Autodesk Inventor part; units mm, degrees
ref_plane "Work Plane1" through (0, 5, 0) normal (0, 1, 0) x (1, 0, 0)
ref_plane "Work Plane3" through (0, 15.4, 0) normal (0, 1, 0) x (1, 0, 0)
ref_plane "YZ Plane" through (0, 0, 0) normal (1, 0, 0) x (0, 1, 0)
sketch "Sketch1" plane through (0, 0, 0) normal (0, 1, 0) x (-1, 0, 0)
  circle A0 centre (0, 0) radius 88.9
  dimension "d0" = 177.8
extrude "Extrusion1" add sketch "Sketch1" along normal blind 25.4
sketch "Sketch2" plane through (0, 25.4, 0) normal (0, 1, 0) x (1, 0, 0)
  circle A0 centre (0, 0) radius 87.4
  line L0 (0, 0) -> (-10.8342, 88.2374)
  circle A1 centre (0, 0) radius 88.9
  line L1 (0, 0) -> (10.8342, 88.2374)
  circle A2 centre (0, 0) radius 34.925
  line L2 (0, 0) -> (0, 88.9)
  circle A3 centre (0, 0) radius 41.275
  point P0 (-4.2563, 34.6647)
  point P1 (4.2563, 34.6647)
  point P2 (10.6514, 86.7485)
  point P3 (-10.6514, 86.7485)
  point P4 (-5.0302, 40.9673)
  point P5 (5.0302, 40.9673)
  dimension "d3" = 174.8
  dimension "d4" = 69.85
  dimension "d10" = 14
  dimension "d11" = 7
  dimension "d45" = 82.55
extrude "Extrusion2" cut sketch "Sketch2" against normal blind 25.4 contours L1 A3 L2 A0 | A0 L2 A3 L0
pattern_circular "Circular Pattern1" count 22 over 360 about axis through (0, 0, 0) along (0, 1, 0) of "Extrusion2"
sketch "Sketch4" plane through (0, 25.4, 0) normal (0, 1, 0) x (1, 0, 0)
  circle A0 centre (0, 0) radius 32.425
  dimension "d16" = 64.85
extrude "Extrusion3" cut sketch "Sketch4" against normal blind 20.4
ref_plane "Work Plane1" through (0, 5, 0) normal (0, 1, 0) x (1, 0, 0)
sketch "Sketch5" plane through (0, 5, 0) normal (0, 1, 0) x (1, 0, 0)
  line L0 (0, 0) -> (0, 25)
  line L1 (0, 0) -> (-25, 0)
  line L2 (0, 0) -> (0, -25)
  line L3 (0, 0) -> (25, 0)
  line L4 (25, 0) -> (25, -9)
  line L5 (0, -25) -> (9, -25)
  line L6 (9, -25) -> (9, -9)
  line L7 (9, -9) -> (25, -9)
  line L8 (0, -25) -> (-9, -25)
  line L9 (-9, -25) -> (-9, -9)
  line L10 (-9, -9) -> (-25, -9)
  line L11 (-25, -9) -> (-25, 0)
  line L12 (-25, 0) -> (-25, 9)
  line L13 (-25, 9) -> (-9, 9)
  line L14 (-9, 9) -> (-9, 25)
  line L15 (-9, 25) -> (0, 25)
  line L16 (9, 25) -> (0, 25)
  line L17 (9, 25) -> (9, 9)
  line L18 (9, 9) -> (25, 9)
  line L19 (25, 9) -> (25, 0)
  dimension "d65" = 25
  dimension "d66" = 25
  dimension "d67" = 25
  dimension "d68" = 25
  dimension "d69" = 9
  dimension "d70" = 9
  dimension "d71" = 9
  dimension "d72" = 9
  dimension "d85" = 9
  dimension "d86" = 9
  dimension "d87" = 9
  dimension "d88" = 9
extrude "Extrusion4" add sketch "Sketch5" along normal blind 15
ref_plane "Work Plane3" through (0, 15.4, 0) normal (0, 1, 0) x (1, 0, 0)
sketch "Sketch21" plane through (0, 25.4, 0) normal (0, 1, 0) x (1, 0, 0)
  circle A0 centre (0, 0) radius 32.425
  circle A1 centre (0, 0) radius 37.425
  dimension "d51" = 64.85
  dimension "d52" = 74.85
extrude "Extrusion8" cut sketch "Sketch21" against normal blind 2
sketch "Sketch23" plane through (0, 0, 0) normal (0, -1, 0) x (1, 0, 0)
  circle A0 centre (0, 0) radius 11
  dimension "d60" = 22
extrude "Extrusion10" cut sketch "Sketch23" against normal blind 7
sketch "Sketch7" plane through (0, 15.4, 0) normal (0, 1, 0) x (1, 0, 0)
  line L0 (-6, 6) -> (6, 6)
  line L1 (6, 6) -> (6, -6)
  line L2 (6, -6) -> (-6, -6)
  line L3 (-6, -6) -> (-6, 6)
  line L4 (-15, 15) -> (15, 15)
  line L5 (15, 15) -> (15, -15)
  line L6 (-15, -15) -> (-15, 15)
  line L7 (15, -15) -> (-15, -15)
  point P0 (0, 0)
  dimension "d32" = 9
  dimension "d33" = 9
  dimension "d34" = 9
  dimension "d35" = 9
extrude "Extrusion6" cut sketch "Sketch7" against normal blind 5 contours L0 L1 L2 L3
sketch "Sketch25" plane through (0, 20, 0) normal (0, 1, 0) x (1, 0, 0)
  line L0 (-22, 6) -> (-6, 6)
  line L1 (-6, 6) -> (-6, 22)
  line L2 (-6, 22) -> (6, 22)
  line L3 (6, 22) -> (6, 6)
  line L4 (6, 6) -> (22, 6)
  line L5 (22, 6) -> (22, -6)
  line L6 (22, -6) -> (6, -6)
  line L7 (6, -6) -> (6, -22)
  line L8 (6, -22) -> (-6, -22)
  line L9 (-6, -22) -> (-6, -6)
  line L10 (-22, -6) -> (-6, -6)
  line L11 (-22, -6) -> (-22, 6)
  line L12 (-9, 25) -> (-9, 9)
  line L13 (9, 25) -> (-9, 25)
  line L14 (9, 9) -> (9, 25)
  line L15 (9, 9) -> (25, 9)
  line L16 (9, -9) -> (25, -9)
  line L17 (25, -9) -> (25, 9)
  line L18 (9, -25) -> (9, -9)
  line L19 (-9, -25) -> (9, -25)
  line L20 (-9, -9) -> (-9, -25)
  line L21 (-25, -9) -> (-9, -9)
  line L22 (-25, 9) -> (-25, -9)
  line L23 (-9, 9) -> (-25, 9)
  point P0 (0, 0)
  dimension "d73" = 3
  dimension "d74" = 3
  dimension "d75" = 3
  dimension "d76" = 3
  dimension "d77" = 3
  dimension "d78" = 3
  dimension "d79" = 3
  dimension "d80" = 3
  dimension "d81" = 3
  dimension "d82" = 3
  dimension "d83" = 3
  dimension "d84" = 3
extrude "Extrusion11" cut sketch "Sketch25" against normal blind 5 contours L0 L1 L2 L3 L4 L5 L6 L7 L8 L9 L10 L11
sketch "Sketch27" plane through (0, 25.4, 0) normal (0, 1, 0) x (1, 0, 0)
  circle A0 centre (0, 0) radius 88.9
  line L0 (-88.9, 0) -> (88.9, 0)
ref_plane "Work Plane4" through (-88.9, 25.4, 0) normal (0, 0, 1) x (1, 0, 0)
sketch "Sketch28" plane through (-88.9, 25.4, 0) normal (0, 0, 1) x (1, 0, 0)
  line L0 (-17.5989, 18.4525) -> (205.1439, 18.4525)
  line L1 (205.1439, 18.4525) -> (205.1439, -42.1057)
  line L2 (205.1439, -42.1057) -> (-17.5989, -42.1057)
  line L3 (-17.5989, -42.1057) -> (-17.5989, 18.4525)
  point P0 (88.9, -25.4)
extrude "Extrusion12" cut sketch "Sketch28" along normal through all
equation "\"d11\" = 0.5 * d10"
equation "\"d33\" = d32"
equation "\"d34\" = d32"
equation "\"d35\" = d32"
equation "\"d75\" = d73"
equation "\"d76\" = d73"
equation "\"d77\" = d73"
equation "\"d78\" = d73"
equation "\"d80\" = d73"
equation "\"d83\" = d73"
properties part number "Capsule_Design_Final"
Build history of the part. All positions in model axes, mm. A direction names the side the tool comes from. Coordinates: 2 decimals unless noted, no trailing zeros. Order: outer loops, then holes, each group sorted by start corner. A loop starts at its lowest first (then second) coordinate and runs counter-clockwise, first axis right, second up. Notation, with made-up numbers: (29, 22) - (37, 22) arc R13 cw to (37, 30) - close; hole circle Ø2 at (57, -25). An arc over 180 degrees is marked (long way). Write item = value, one per line. Start each with the question number.
1) Saw through at B-B on x = -43. Write the cut outline in (y, z), then the cut area to 3 significant figures.
2) Wall check: line 1 along Z through (x, y) = (76, 11); line 2 along Z through (x, y) = (-34, 1); line 3 along Z through (x, y) = (72, 10.5). Give the ranges that are in metal, low to high. Write a range as from..to.
3) Saw through at D-D on x = 61. Write the cut outline in (y, z).
4) Flat gauge pins, fed straight in: pin 1 Ø6 at (x, y) = (-47.5, 20) entering from -Z; pin 2 Ø3 at (x, z) = (15.5, -3) entering from +Y; pin 3 Ø1.5 at (x, z) = (56.5, -31.5) entering from -Y; pin 4 Ø4 at (x, y) = (-2, 18.5) entering from +Z. Where does each tip first touch, or does it go through?
5) Saw through at A-A on x = 0. Write the cut outline in (y, z) (3 decimals), then the cut area to 3 significant figures.
6) 3-axis set-ups, long thin cutter, end or side, ignore diameter. For faces 1 (the face through (0, 7, -4)), 2 (the face through (6, 13, -3)), 3 (the face through (10.415, 12.878, -63.162)), 4 (the face through (0, 12, -25)): which of +Z, -Z, +X, -X, +Y, -Y reach the whole face in a straight line?
7) Saw through at C-C on y = 2.5. Count the separate pieces of the cut face and the enclosed holes in it, then the cut area to 3 significant figures.
From the geometry:
q1.outline = (0, -77.81) - (25.4, -77.81) - (25.4, -76.09) - (0, -76.09) - close; (0, -51.74) - (25.4, -51.74) - (25.4, -47.6) - (0, -47.6) - close; (0, -28.9) - (25.4, -28.9) - (25.4, -26.4) - (0, -26.4) - close; (0, -13.6) - (25.4, -13.6) - (25.4, -11.67) - (0, -11.67) - close; (0, -0.89) - (25.4, -0.89) - (25.4, 0) - (0, 0) - close
q1.area = 284 mm^2
q2.line_1 = -46.12..-43.16, -24.03..-20.62, -1.57..0
q2.line_2 = -82.14..-80.52, -78.71..-70.56, -40.91..-37.64, -23.4..0
q2.line_3 = -52.15..-49.55, -48.4..-44.2, -22.76..-19.54, -1.49..0
q3.outline = (0, -64.67) - (25.4, -64.67) - (25.4, -62.59) - (0, -62.59) - close; (0, -41) - (25.4, -41) - (25.4, -37.45) - (0, -37.45) - close; (0, -19.29) - (25.4, -19.29) - (25.4, -16.55) - (0, -16.55) - close; (0, -1.26) - (25.4, -1.26) - (25.4, 0) - (0, 0) - close
q4.pin_1 = -76.96
q4.pin_2 = 15
q4.pin_3 = through
q4.pin_4 = -22
q5.outline = (0, -88.9) - (25.4, -88.9) - (25.4, -87.4) - (0, -87.4) - close; (0, -41.275) - (25.4, -41.275) - (25.4, -37.425) - (23.4, -37.425) - (23.4, -32.425) - (5, -32.425) - (5, -25) - (20, -25) - (20, -22) - (15, -22) - (15, -6) - (10.4, -6) - (10.4, 0) - (7, 0) - (7, -11) - (0, -11) - close
q5.area = 575 mm^2
q6.face_1 = +Z, -Y
q6.face_2 = +Z, +Y
q6.face_3 = +Y, -Y
q6.face_4 = +Y
q7.separate_pieces = 1
q7.enclosed_holes = 11
q7.area = 4,250 mm^2
